The listing builds one solid part. Answer for the finished solid, in the listing's coordinates (mm). Face numbers are marked on the shaded views. A direction names the side the tool comes from. Give positions to 0.01 mm unless a question says otherwise; leave off trailing zeros. Write each loop counter-clockwise with the first axis right and the second up, starting at its lowest first coordinate (ties: lowest second). Pieces come first, ordered by that corner, then holes. Notation, with made-up numbers: (41.5, -38.5) - (49.5, -38.5) arc R28 cw to (49.5, -6.5) - close; hole circle Ø6 at (72.25, 87.5). An arc over 180 degrees is marked (long way). Return JSON: item names as keys, results as strings.
from build123d import *

# Parameters (mm, degrees)
CHAMFER1_SIZE = 0.1
CHAMFER2_SIZE = 0.1


with BuildPart() as part:
    # Sketch2 → Revolve1 (revolve)
    with BuildSketch(Plane.XY):
        Polygon((6.945, -1.55), (6.945, 1.55), (7.9875, 1.55), (7.9875, 6.35), (11, 6.35), (11, 4.75), (8.75, 4.75), (8.75, -4.75), (11, -4.75), (11, -6.35), (7.9875, -6.35), (7.9875, -1.55), align=None)
    revolve(axis=Axis((0, 30.498149714, 0), (0, -1, 0)))

    # Chamfer1
    chamfer1_edges = [part.edges().sort_by_distance(p)[0] for p in [
        (-7.9875, 6.35, 0),
    ]]
    chamfer(chamfer1_edges, length=CHAMFER1_SIZE)

    # Chamfer2
    chamfer2_edges = [part.edges().sort_by_distance(p)[0] for p in [
        (-7.9875, -6.35, 0),
    ]]
    chamfer(chamfer2_edges, length=CHAMFER2_SIZE)


solid = part.part
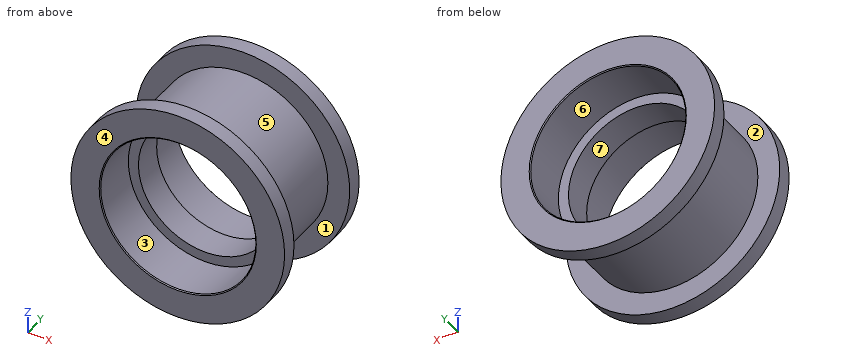
Item 1: A cutting plane is placed at D-D on z = 9.75. Determine the outline of the cut face in (x, y).
Answer below:
{"outline": "(-5.09, -6.35) - (5.09, -6.35) - (5.09, -4.75) - (-5.09, -4.75) - close; (-5.09, 4.75) - (5.09, 4.75) - (5.09, 6.35) - (-5.09, 6.35) - close"}
Item 2: Consider L1, parallel to Y at x = 6.25, z = 9; L2, parallel to Z at x = 0, y = 3.7; L3, parallel to Z at x = 0, y = 0.1 (3 decimals). Determine where each line is inside the solid, lowest interval first.
Answer below:
{"L1": "y = -6.35 to -4.75, 4.75 to 6.35", "L2": "z = -8.75 to -7.99, 7.99 to 8.75", "L3": "z = -8.75 to -6.945, 6.945 to 8.75"}
Item 3: For the marked faces 5, 6 and 7, determine the directions among +Z, -Z, +X, -X, +Y, -Y from which every point of the face is accessible in a straight line to the end or side of a thin tool.
Answer below:
{"face 5": "none", "face 6": "+Y", "face 7": "+Y, -Y"}
Item 4: The mould has two halves that part along Y. Classify the marked faces 1, 2, 3 and 4: +Y half, -Y half, draft (parallel to the pull), parting line (faces both ways), or undercut.
Answer below:
{"face 1": "undercut", "face 2": "undercut", "face 3": "draft", "face 4": "-Y half"}
Item 5: Flat-ended cylindrical pins translate along their axes: P1, Ø4, axis at y = 4, z = 6.5, coming from the +X side; P2, Ø4, axis at x = -8.5, y = -3.5, coming from the -Z side; P3, Ø1, axis at y = -4, z = 1.5, coming from the -X side; P4, Ø12.5, axis at x = 0, z = 0, coming from the -Y side. Find the tip coordinate at first contact, or state that the pin passes through.
Answer below:
{"P1": "stops at x = 9.97", "P2": "stops at z = -8.54", "P3": "stops at x = -8.69", "P4": "passes through"}
